```python
from build123d import *

# Parameters (mm, degrees)
F0_R          = 8.1
F0_R_2        = 5.1
F1_DEPTH      = 17.97
F4_DEPTH      = 7.6
F4_DEPTH_BACK = 0.4
F6_DEPTH      = 5


with BuildPart() as f1:
    # F0 (on Top) → F1 (new body)
    with BuildSketch(Plane.XY):
        Circle(F0_R)
        Circle(F0_R_2, mode=Mode.SUBTRACT)
    extrude(amount=F1_DEPTH)

    # F3 (on offset) → F4 (cut, two sides)
    with BuildSketch(Plane.XZ.offset(-9.09)) as f4_sk:
        Polygon((4.6, 0), (4.6, 17.97), (0, 17.97), (-4.6, 17.97), (-4.6, 0), (0, 0), align=None)
    extrude(amount=F4_DEPTH, mode=Mode.SUBTRACT)
    extrude(f4_sk.sketch, amount=-F4_DEPTH_BACK, mode=Mode.SUBTRACT)

    # F5 (on face) → F6 (join)
    with BuildSketch(Plane(origin=(0, 0, 0), x_dir=(1, 0, 0), z_dir=(0, 0, -1))):
        Polygon((0, 5.044552), (-0.75, 5.044552), (-0.75, 3.444552), (0, 3.444552), (0.75, 3.444552), (0.75, 5.044552), align=None)
        with BuildLine():
            ThreePointArc((0.75, 5.044552), (0, 5.1), (-0.75, 5.044552))
            Line((-0.75, 5.044552), (0, 5.044552))
            Line((0, 5.044552), (0.75, 5.044552))
        make_face()
    extrude(amount=-F6_DEPTH)


solid = f1.part
```
Work out the finished part from the listing and answer in its coordinate system (mm). A direction names the side the tool comes from. Coordinates: 2 decimals unless noted, no trailing zeros. Loops run counter-clockwise (first coordinate to the right, second up) from the corner with the lowest first, then second, coordinate; pieces in that order, holes last.
1) Consider probe 1 along X at (y, z) = (0, 10.5); probe 2 along Y at (x, z) = (-0.25, 14); probe 3 along X at (y, z) = (-4, 8.5). Determine where each line is inside the solid, lowest interval first.
Results:
probe 1: x = -8.1 to -5.1, 5.1 to 8.1
probe 2: y = -8.1 to -5.09
probe 3: x = -7.04 to -3.16, 3.16 to 7.04
2) Section C-C (y = 3.25) is taken. Give the vertices of the cut face in (x, z).
Results:
outline: (-7.42, 0) - (-4.6, 0) - (-4.6, 17.97) - (-7.42, 17.97) - close; (4.6, 0) - (7.42, 0) - (7.42, 17.97) - (4.6, 17.97) - close
3) Section D-D (z = 12) is taken. Give the vertices of the cut face in (x, y).
Results:
outline: (-4.6, 2.2) - (-4.6, 6.67) arc R8.1 ccw (long way) to (4.6, 6.67) - (4.6, 2.2) arc R5.1 cw (long way) to start
4) Section A-A (y = 0) is taken. Give the vertices of the cut face in (x, z), plus the area to 3 significant figures.
Results:
outline: (-8.1, 0) - (-5.1, 0) - (-5.1, 17.97) - (-8.1, 17.97) - close; (5.1, 0) - (8.1, 0) - (8.1, 17.97) - (5.1, 17.97) - close
area: 108 mm2
5) Flat-ended cylindrical pins translate along their axes: pin 1 (1.6 mm diameter, centred on x = 0, y = -4, fed in from +Z); pin 2 (1.8 mm diameter, centred on y = -4, z = 2.5, fed in from +X); pin 3 (5 mm diameter, centred on y = 3.5, z = 12.5, fed in from -X); pin 4 (1.5 mm diameter, centred on x = 3.5, y = -0.5, fed in from +Z). Find the tip coordinate at first contact, or state that the pin passes through.
Results:
pin 1: stops at z = 5
pin 2: stops at x = 7.48
pin 3: stops at x = -8.04
pin 4: passes through
6) For faces 4 (the flat face through (0, -6, 17.97)), 5 (the flat face through (0, -4, 5)), 6 (the flat face through (4.6, 4, 9)), determine the directions among +Z, -Z, +X, -X, +Y, -Y from which every point of the face is accessible in a straight line to the end or side of a thin tool.
Results:
face 4: +Z, +X, -X, +Y, -Y
face 5: +Z, +Y
face 6: +Z, -Z, +Y
7) For a pull along Y with two mould halves and no side action, classify faces 1 (the flat face through (-0.75, -4, 2)), 2 (the cylindrical face through (-0.1, -5.1, 8.9)), 3 (the flat face through (0, -3.445, 2)) as +Y half, -Y half, draft (parallel to the pull), parting line (faces both ways), or undercut.
Results:
face 1: draft
face 2: undercut
face 3: +Y half
8) Section B-B (x = 0) is taken. Give the vertices of the cut face in (y, z).
Results:
outline: (-8.1, 0) - (-3.44, 0) - (-3.44, 5) - (-5.1, 5) - (-5.1, 17.97) - (-8.1, 17.97) - close
